Geometry check sheet. Reference: the model listing, model coordinates, mm. A direction names the side the tool comes from. Round coordinates to 2 decimals unless told otherwise and drop trailing zeros. Write each loop counter-clockwise with the first axis right and the second up, starting at its lowest first coordinate (ties: lowest second). Pieces come first, ordered by that corner, then holes. Notation, with made-up numbers: M 31.5,25 L 53.5,25 A19 cw 53.5,37 Z; hole C -32,17.5 d3. An arc over 180 degrees is marked long. Answer in a Markdown table with one row per item. Add a question column.
from build123d import *

# Parameters (mm, degrees)
SKETCH_1_R                   = 106
EXTRUDE_1_DEPTH              = 98
SKETCH_2_R                   = 82.5
CUT_EXTRUDE_1_DEPTH          = 5
PATTERN_CIRCULAR_1_COUNT     = 3
HOLE_WIZARD_M10_2_AT_2_COUNT = 2
HOLE_WIZARD_M10_2_AT_2_PITCH = 25
PATTERN_CIRCULAR_2_COUNT     = 3


with BuildPart() as part:
    # 草图1 → 凸台-拉伸1 (new body)
    with BuildSketch(Plane.XY):
        Circle(SKETCH_1_R)
    extrude(amount=EXTRUDE_1_DEPTH)

    # 草图2 → 切除-拉伸1 (cut)
    with BuildSketch(Plane.XY.offset(98)):
        Circle(SKETCH_2_R)
    extrude(amount=-CUT_EXTRUDE_1_DEPTH, mode=Mode.SUBTRACT)

    # 草图3 → M10 螺纹孔1 (revolve, cut)
    with BuildSketch(Plane(origin=(0, 90, 98), x_dir=(0, -1, 0), z_dir=(1, 0, 0))):
        Polygon((0, 0), (0, 32.553657631), (4.25, 30), (4.25, 0), align=None)
    hole_wizard_m10_1 = revolve(axis=Axis((0, 90, 104.35), (0, 0, -1)), mode=Mode.SUBTRACT)

    # 阵列(圆周)1: M10 螺纹孔1 ×3 about axis
    pattern_circular_1_axis = Axis((0, 0, 0), (0, 0, 1))
    for i in range(1, PATTERN_CIRCULAR_1_COUNT):
        add(hole_wizard_m10_1.rotate(pattern_circular_1_axis, i * 360 / PATTERN_CIRCULAR_1_COUNT), mode=Mode.SUBTRACT)

    # 草图5 → M10 螺纹孔2 (revolve, cut)
    with BuildSketch(Plane(origin=(0, 100, 0), x_dir=(0, 1, 0), z_dir=(1, 0, 0))):
        Polygon((0, 0), (0, 27.053657631), (4.25, 24.5), (4.25, 0), align=None)
    hole_wizard_m10_2 = revolve(axis=Axis((0, 100, -6.35), (0, 0, 1)), mode=Mode.SUBTRACT)

    # M10 螺纹孔2 at 2: M10 螺纹孔2 ×2
    with Locations(*[(0, -i * HOLE_WIZARD_M10_2_AT_2_PITCH, 0) for i in range(1, HOLE_WIZARD_M10_2_AT_2_COUNT)]):
        add(hole_wizard_m10_2, mode=Mode.SUBTRACT)

    # 阵列(圆周)2: M10 螺纹孔2 ×3 about axis
    pattern_circular_2_axis = Axis((0, 0, 0), (0, 0, 1))
    for i in range(1, PATTERN_CIRCULAR_2_COUNT):
        add(hole_wizard_m10_2.rotate(pattern_circular_2_axis, i * 360 / PATTERN_CIRCULAR_2_COUNT), mode=Mode.SUBTRACT)

    # 阵列(圆周)2 copy 1 sketch → 阵列(圆周)2 copy 1 (revolve, cut)
    with BuildSketch(Plane(origin=(-64.951905284, -37.5, 0), x_dir=(-0.8660254037844387, -0.4999999999999998, 0), z_dir=(-0.4999999999999998, 0.8660254037844387, 0))):
        Polygon((0, 0), (0, 27.053657631), (4.25, 24.5), (4.25, 0), align=None)
    revolve(axis=Axis((-64.951905284, -37.5, -6.35), (0, 0, 1)), mode=Mode.SUBTRACT)

    # 阵列(圆周)2 copy 2 sketch → 阵列(圆周)2 copy 2 (revolve, cut)
    with BuildSketch(Plane(origin=(64.951905284, -37.5, 0), x_dir=(0.8660254037844384, -0.5000000000000004, 0), z_dir=(-0.5000000000000004, -0.8660254037844384, 0))):
        Polygon((0, 0), (0, 27.053657631), (4.25, 24.5), (4.25, 0), align=None)
    revolve(axis=Axis((64.951905284, -37.5, -6.35), (0, 0, 1)), mode=Mode.SUBTRACT)


solid = part.part
Item 1: Section check C-C, the plane z = 52. Record the boundary of the cut face in (x, y), and give its area (3 significant figures).
Item 2: Section check A-A, the plane y = 0. Record the boundary of the cut face in (x, z), and give its area (3 significant figures).
Item 3: Access from +Z, -Z, +X, -X, +Y, -Y to the whole of each face (thin tool, end or side, straight path). Record for faces 1 (the cylindrical face through (-17.88, -80.54, 95.54)), 2 (the flat face through (54.5, -62.3, 98)), 3 (the cylindrical face through (-1.277, 79.054, 12.078)).
Item 4: Section check B-B, the plane x = -54.5. Record the boundary of the cut face in (y, z), and give its area (3 significant figures).
Item 5: Scan lines: probe 1 along X at (y, z) = (-45, 75); probe 2 along X at (y, z) = (-37, 10); probe 3 along Y at (x, z) = (-1.5, 34.5). Record each from-to range of solid material in increasing order. Write a range as from..to.
Item 6: Mould release check, pull along X, two halves, no side actions. Record for faces 4 (the cylindrical face through (56.985, 89.38, 48.314)), 5 (the conical face through (-0.03, 99.26, 26.61)), 6 (the flat face through (-1, 1, 0)), 7 (the cylindrical face through (61.368, -35.215, 12.078)): +X half, -X half, draft (parallel to the pull), parting line (faces both ways), or undercut.
Item 7: Gauge pin test, flat ends, axial feed: pin 1 Ø5 at (x, y) = (-64.95, -37.5) entering from -Z; pin 2 Ø4 at (x, z) = (65, 69) entering from -Y; pin 3 Ø11 at (x, y) = (64.95, -37.5) entering from +Z. Record the tip position at first contact, or that the pin passes through.
Result sheet:
| question | item | result |
|---|---|---|
| 1 | outline | C 0,0 d212 |
| 1 | area | 35,300 mm^2 |
| 2 | outline | M -106,0 L 106,0 L 106,98 L 82.5,98 L 82.5,93 L -82.5,93 L -82.5,98 L -106,98 Z |
| 2 | area | 20,000 mm^2 |
| 3 | face 1 | +Z |
| 3 | face 2 | +Z, +X, -X, +Y, -Y |
| 3 | face 3 | -Z |
| 4 | outline | M -90.92,0 L 90.92,0 L 90.92,98 L 61.94,98 L 61.94,93 L -61.94,93 L -61.94,98 L -90.92,98 Z |
| 4 | area | 17,200 mm^2 |
| 5 | probe 1 | x = -95.97..-82.19, -73.69..73.69, 82.19..95.97 |
| 5 | probe 2 | x = -99.33..-69.17, -60.73..60.73, 69.17..99.33 |
| 5 | probe 3 | y = -105.99..105.99 |
| 6 | face 4 | parting line |
| 6 | face 5 | undercut |
| 6 | face 6 | draft |
| 6 | face 7 | undercut |
| 7 | pin 1 | stops at z = 25.55 |
| 7 | pin 2 | stops at y = -85.25 |
| 7 | pin 3 | stops at z = 93 |
